```python
from build123d import *

# Parameters (mm, degrees)
ESTRUSIONE_ESTRUSIONE1_DEPTH = 140
FORO_6_5_6_5_1_D             = 6.5
FORO_6_5_6_5_2_D             = 6.5
FORO_6_5_6_5_2_DEPTH         = 5
FORO_6_5_6_5_2_TIP           = 1.952797012
TAGLIO_ESTRUSIONE3_REACH     = 52
SCHIZZO10_R                  = 7
TAGLIO_ESTRUSIONE6_REACH     = 52
SCHIZZO13_R                  = 6.5
SMUSSO1_SIZE                 = 3
M3_5_CLEARANCE_HOLE1_D       = 3.9
M3_5_CLEARANCE_HOLE2_D       = 3.9


with BuildPart() as part:
    # Schizzo1 → Estrusione-Estrusione1 (new body)
    with BuildSketch(Plane.XY):
        Polygon((0, 0), (0, 50), (5, 50), (5, 5), (50, 5), (50, 0), align=None)
    extrude(amount=ESTRUSIONE_ESTRUSIONE1_DEPTH)

    # Foro Ø6.5 (6.5)-1 (through all)
    with Locations(Plane(origin=(0, 0, 0), x_dir=(-1, 0, 0), z_dir=(0, -1, 0))):
        with Locations((-17, -132), (-42, -132)):
            foro_6_5_6_5_1 = Hole(FORO_6_5_6_5_1_D / 2)

    # Foro Ø6.5 (6.5)-2
    with Locations(Plane.ZY):
        with Locations((132, 42), (132, 17)):
            Hole(FORO_6_5_6_5_2_D / 2, depth=FORO_6_5_6_5_2_DEPTH)
            with Locations((0, 0, -(FORO_6_5_6_5_2_DEPTH + FORO_6_5_6_5_2_TIP / 2))):  # 118° drill point
                Cone(0, FORO_6_5_6_5_2_D / 2, FORO_6_5_6_5_2_TIP, mode=Mode.SUBTRACT)

    # Specchia1: Foro Ø6.5 (6.5)-1 across plane
    add(foro_6_5_6_5_1.mirror(Plane.XY.offset(70)), mode=Mode.SUBTRACT)

    # Schizzo10 → Taglio-Estrusione3 (cut, up to next)
    with BuildSketch(Plane.ZY, mode=Mode.PRIVATE) as taglio_estrusione3_sk1:
        with Locations((80, 30)):
            Circle(SCHIZZO10_R)
    taglio_estrusione3_tool1 = extrude(taglio_estrusione3_sk1.sketch, amount=-TAGLIO_ESTRUSIONE3_REACH, mode=Mode.PRIVATE) & part.part
    add(taglio_estrusione3_tool1.solids().sort_by_distance((0, 30, 80))[0], mode=Mode.SUBTRACT)

    # Schizzo13 → Taglio-Estrusione6 (cut, up to next)
    with BuildSketch(Plane.ZY, mode=Mode.PRIVATE) as taglio_estrusione6_sk1:
        with Locations((35.178130338, 26)):
            Circle(SCHIZZO13_R)
    taglio_estrusione6_tool1 = extrude(taglio_estrusione6_sk1.sketch, amount=-TAGLIO_ESTRUSIONE6_REACH, mode=Mode.PRIVATE) & part.part
    add(taglio_estrusione6_tool1.solids().sort_by_distance((0, 26, 35.17813))[0], mode=Mode.SUBTRACT)
    # Schizzo13 → Taglio-Estrusione6 (cut, up to next)
    with BuildSketch(Plane.ZY, mode=Mode.PRIVATE) as taglio_estrusione6_sk2:
        with BuildLine():
            Line((18.178130338, 43.25), (21.178130338, 43.25))
            ThreePointArc((21.178130338, 43.25), (22.928130338, 41.5), (21.178130338, 39.75))
            Line((21.178130338, 39.75), (18.178130338, 39.75))
            ThreePointArc((18.178130338, 39.75), (16.428130338, 41.5), (18.178130338, 43.25))
        make_face()
    taglio_estrusione6_tool2 = extrude(taglio_estrusione6_sk2.sketch, amount=-TAGLIO_ESTRUSIONE6_REACH, mode=Mode.PRIVATE) & part.part
    add(taglio_estrusione6_tool2.solids().sort_by_distance((0, 41.5, 19.67813))[0], mode=Mode.SUBTRACT)
    # Schizzo13 → Taglio-Estrusione6 (cut, up to next)
    with BuildSketch(Plane.ZY, mode=Mode.PRIVATE) as taglio_estrusione6_sk3:
        with BuildLine():
            Line((18.178130338, 8.75), (21.178130338, 8.75))
            ThreePointArc((21.178130338, 8.75), (22.928130338, 10.5), (21.178130338, 12.25))
            Line((21.178130338, 12.25), (18.178130338, 12.25))
            ThreePointArc((18.178130338, 12.25), (16.428130338, 10.5), (18.178130338, 8.75))
        make_face()
    taglio_estrusione6_tool3 = extrude(taglio_estrusione6_sk3.sketch, amount=-TAGLIO_ESTRUSIONE6_REACH, mode=Mode.PRIVATE) & part.part
    add(taglio_estrusione6_tool3.solids().sort_by_distance((0, 10.5, 19.67813))[0], mode=Mode.SUBTRACT)
    # Schizzo13 → Taglio-Estrusione6 (cut, up to next)
    with BuildSketch(Plane.ZY, mode=Mode.PRIVATE) as taglio_estrusione6_sk4:
        with BuildLine():
            Line((52.178130338, 43.25), (49.178130338, 43.25))
            ThreePointArc((49.178130338, 43.25), (47.428130338, 41.5), (49.178130338, 39.75))
            Line((49.178130338, 39.75), (52.178130338, 39.75))
            ThreePointArc((52.178130338, 39.75), (53.928130338, 41.5), (52.178130338, 43.25))
        make_face()
    taglio_estrusione6_tool4 = extrude(taglio_estrusione6_sk4.sketch, amount=-TAGLIO_ESTRUSIONE6_REACH, mode=Mode.PRIVATE) & part.part
    add(taglio_estrusione6_tool4.solids().sort_by_distance((0, 41.5, 50.67813))[0], mode=Mode.SUBTRACT)
    # Schizzo13 → Taglio-Estrusione6 (cut, up to next)
    with BuildSketch(Plane.ZY, mode=Mode.PRIVATE) as taglio_estrusione6_sk5:
        with BuildLine():
            Line((52.178130338, 8.75), (49.178130338, 8.75))
            ThreePointArc((49.178130338, 8.75), (47.428130338, 10.5), (49.178130338, 12.25))
            Line((49.178130338, 12.25), (52.178130338, 12.25))
            ThreePointArc((52.178130338, 12.25), (53.928130338, 10.5), (52.178130338, 8.75))
        make_face()
    taglio_estrusione6_tool5 = extrude(taglio_estrusione6_sk5.sketch, amount=-TAGLIO_ESTRUSIONE6_REACH, mode=Mode.PRIVATE) & part.part
    add(taglio_estrusione6_tool5.solids().sort_by_distance((0, 10.5, 50.67813))[0], mode=Mode.SUBTRACT)

    # Smusso1
    smusso1_edges = [part.edges().sort_by_distance(p)[0] for p in [
        (2.5, 50, 140),
        (2.5, 50, 0),
        (50, 2.5, 140),
        (50, 2.5, 0),
    ]]
    chamfer(smusso1_edges, length=SMUSSO1_SIZE)

    # M3.5 Clearance Hole1 (through all)
    with Locations(Plane(origin=(0, 40, 70), x_dir=(0, 0, -1), z_dir=(-1, 0, 0))):
        with Locations((0, 0), (-20, 0), (-20, 20), (0, 20)):
            Hole(M3_5_CLEARANCE_HOLE1_D / 2)

    # M3.5 Clearance Hole2 (through all)
    with Locations(Plane(origin=(20, 0, 110), x_dir=(-1, 0, 0), z_dir=(0, -1, 0))):
        with Locations((0, 0), (-20, 0), (-20, 20), (0, 20)):
            Hole(M3_5_CLEARANCE_HOLE2_D / 2)


solid = part.part
```
Geometry check sheet. Reference: the model listing, model coordinates, mm. A direction names the side the tool comes from. Coordinates: 2 decimals unless noted, no trailing zeros. Loops run counter-clockwise (first coordinate to the right, second up) from the corner with the lowest first, then second, coordinate; pieces in that order, holes last. Notation, with made-up numbers: (-23, 34.5) - (11, 34.5) arc R17 ccw to (11, 53.5) - close; hole circle Ø6 at (-21, -15). An arc over 180 degrees is marked (long way). One line per item, written item: value. Start each with the question number.
(1) Cross-section at A-A on z = 8. Enter the section's corners in (x, y).
(2) Depth check by flat-ended pin: P1, Ø12, axis at x = 11.5, z = 88.5, coming from the +Y side; P2, Ø4, axis at y = 42, z = 132, coming from the -X side; P3, Ø4.5, axis at y = 20, z = 70, coming from the +X side. Enter the tip coordinate at first touch or a pass-through.
(3) Cross-section at C-C on y = 6.5. Enter the section's corners in (x, z), plus the area to 3 significant figures.
(4) Tool access check on faces 1 (the flat face through (2, 43.25, 51)), 2 (the flat face through (0, 25, 69)). Record the directions out of +Z, -Z, +X, -X, +Y, -Y that give a thin tool (end or side, any length) a straight path to the whole face; none if there is none.
(5) Cross-section at B-B on z = 80. Enter the section's corners in (x, y), plus the area to 3 significant figures.
(6) Mould release check, pull along Z, two halves, no side actions. Record for faces 3 (the cylindrical face through (2.46, 41.54, 47.43)), 4 (the flat face through (50, 3, 69)), 5 (the flat face through (13, 4, 0)): released by +Z, released by -Z, zero draft, split by the parting line, or undercut.
(7) Material ranges on line 1 (Y direction, x = 2.4, z = 132); line 2 (X direction, y = 3.8, z = 110); line 3 (Z direction, x = 17, y = 2.1), recorded low to high. Write a range as [from, to].
Results below:
1. outline: (0, 0) - (13.75, 0) - (13.75, 5) - (5, 5) - (5, 50) - (0, 50) - close; (20.25, 0) - (38.75, 0) - (38.75, 5) - (20.25, 5) - close; (45.25, 0) - (50, 0) - (50, 5) - (45.25, 5) - close
2. P1: stops at y = 5
2. P2: passes through
2. P3: stops at x = 5
3. outline: (0, 0) - (5, 0) - (5, 140) - (0, 140) - close
3. area: 700 mm2
4. face 1: +X, -X
4. face 2: +Z, -Z, -X, +Y, -Y
5. outline: (0, 0) - (50, 0) - (50, 5) - (5, 5) - (5, 23) - (0, 23) - close; (0, 37) - (5, 37) - (5, 50) - (0, 50) - close
5. area: 405 mm2
6. face 3: undercut
6. face 4: zero draft
6. face 5: released by -Z
7. line 1: y = [0, 13.75], [20.25, 38.75], [45.25, 50]
7. line 2: x = [0, 18.05], [21.95, 38.05], [41.95, 50]
7. line 3: z = [0, 4.75], [11.25, 128.75], [135.25, 140]
